Check sheet for the modelled part. Datum: model origin and axes. Units: mm. Face numbers are marked on the shaded views. A direction names the side the tool comes from. Round coordinates to 2 decimals unless told otherwise and drop trailing zeros. Write each loop counter-clockwise with the first axis right and the second up, starting at its lowest first coordinate (ties: lowest second). Pieces come first, ordered by that corner, then holes. Notation, with made-up numbers: (86, 52.5) -> (140, 52.5) arc R17 ccw to (140, 81.5) -> close; hole circle Ø7 at (-3.75, -13.5). An arc over 180 degrees is marked (long way). One line per item, written item: value.
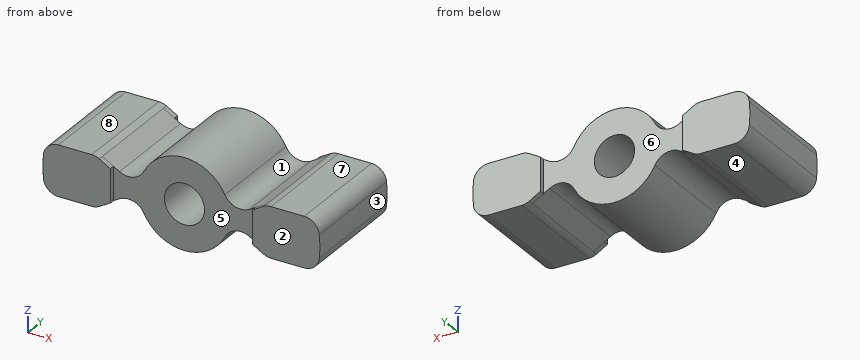
from build123d import *

# Parameters (mm, degrees)
F0_R     = 4
F1_DEPTH = 10
F3_DEPTH = 1


# Not quite as in the source:
# - a pattern or mirror of a feature is missing from the dataset's text; its kind, count and spacing are read off the source's solid


with BuildPart() as f1:
    # F0 (on Front) → F1 (new body, symmetric)
    with BuildSketch(Plane.XZ):
        with BuildLine():
            ThreePointArc((-12.8973712231, -2.6245379145), (-10.1504183848, -2.3006178802), (-8.0261072806, -4.072051316))
            ThreePointArc((-8.0261072806, -4.072051316), (0, -9), (8.0261072806, -4.072051316))
            ThreePointArc((8.0261072806, -4.072051316), (10.1504183848, -2.3006178802), (12.8973712231, -2.6245379145))
            Line((12.8973712231, -2.6245379145), (16.315639824, -4.5980762114))
            ThreePointArc((16.315639824, -4.5980762114), (17.0391826887, -4.8977774789), (17.815639824, -5))
            Line((17.815639824, -5), (24.4182308941, -5))
            ThreePointArc((24.4182308941, -5), (26.4511236757, -4.2062064588), (27.4082183506, -2.2448979592))
            ThreePointArc((27.4082183506, -2.2448979592), (27.5, 0), (27.4082183506, 2.2448979592))
            ThreePointArc((27.4082183506, 2.2448979592), (26.4511236757, 4.2062064588), (24.4182308941, 5))
            Line((24.4182308941, 5), (17.815639824, 5))
            ThreePointArc((17.815639824, 5), (17.0391826887, 4.8977774789), (16.315639824, 4.5980762114))
            Line((16.315639824, 4.5980762114), (12.8973712231, 2.6245379145))
            ThreePointArc((12.8973712231, 2.6245379145), (10.1504183848, 2.3006178802), (8.0261072806, 4.072051316))
            ThreePointArc((8.0261072806, 4.072051316), (0, 9), (-8.0261072806, 4.072051316))
            ThreePointArc((-8.0261072806, 4.072051316), (-10.1504183848, 2.3006178802), (-12.8973712231, 2.6245379145))
            Line((-12.8973712231, 2.6245379145), (-16.315639824, 4.5980762114))
            ThreePointArc((-16.315639824, 4.5980762114), (-17.0391826887, 4.8977774789), (-17.815639824, 5))
            Line((-17.815639824, 5), (-24.4182308941, 5))
            ThreePointArc((-24.4182308941, 5), (-26.4511236757, 4.2062064588), (-27.4082183506, 2.2448979592))
            ThreePointArc((-27.4082183506, 2.2448979592), (-27.5, 0), (-27.4082183506, -2.2448979592))
            ThreePointArc((-27.4082183506, -2.2448979592), (-26.4511236757, -4.2062064588), (-24.4182308941, -5))
            Line((-24.4182308941, -5), (-17.815639824, -5))
            ThreePointArc((-17.815639824, -5), (-17.0391826887, -4.8977774789), (-16.315639824, -4.5980762114))
            Line((-16.315639824, -4.5980762114), (-12.8973712231, -2.6245379145))
        make_face()
        Circle(F0_R, mode=Mode.SUBTRACT)
    extrude(amount=F1_DEPTH, both=True)

    # F2 (on face) → F3 (join)
    with BuildSketch(Plane.XZ.offset(10)):
        with BuildLine():
            Line((-24.4182308941, -5), (-17.815639824, -5))
            ThreePointArc((-17.815639824, -5), (-17.0391826887, -4.8977774789), (-16.315639824, -4.5980762114))
            Line((-16.315639824, -4.5980762114), (-14.1075365245, -3.323227177))
            Line((-14.1075365245, -3.323227177), (-14.1075365245, 3.323227177))
            Line((-14.1075365245, 3.323227177), (-16.315639824, 4.5980762114))
            ThreePointArc((-16.315639824, 4.5980762114), (-17.0391826887, 4.8977774789), (-17.815639824, 5))
            Line((-17.815639824, 5), (-24.4182308941, 5))
            ThreePointArc((-24.4182308941, 5), (-26.4511236757, 4.2062064588), (-27.4082183506, 2.2448979592))
            ThreePointArc((-27.4082183506, 2.2448979592), (-27.5, 0), (-27.4082183506, -2.2448979592))
            ThreePointArc((-27.4082183506, -2.2448979592), (-26.4511236757, -4.2062064588), (-24.4182308941, -5))
        make_face()
        with BuildLine():
            Line((14.1075365245, -3.323227177), (16.315639824, -4.5980762114))
            ThreePointArc((16.315639824, -4.5980762114), (17.0391826887, -4.8977774789), (17.815639824, -5))
            Line((17.815639824, -5), (24.4182308941, -5))
            ThreePointArc((24.4182308941, -5), (26.4511236757, -4.2062064588), (27.4082183506, -2.2448979592))
            ThreePointArc((27.4082183506, -2.2448979592), (27.5, 0), (27.4082183506, 2.2448979592))
            ThreePointArc((27.4082183506, 2.2448979592), (26.4511236757, 4.2062064588), (24.4182308941, 5))
            Line((24.4182308941, 5), (17.815639824, 5))
            ThreePointArc((17.815639824, 5), (17.0391826887, 4.8977774789), (16.315639824, 4.5980762114))
            Line((16.315639824, 4.5980762114), (14.1075365245, 3.323227177))
            Line((14.1075365245, 3.323227177), (14.1075365245, -3.323227177))
        make_face()
    f3 = extrude(amount=F3_DEPTH)

    # F3_copies: F3 across plane
    add(f3.mirror(Plane.ZX))


solid = f1.part
Item 1: Sectioned sample at B-B on z = 0. Enter the section's corners in (x, y).
Answer:
outline: (-27.5, -11) -> (-14.11, -11) -> (-14.11, -10) -> (-4, -10) -> (-4, 10) -> (-14.11, 10) -> (-14.11, 11) -> (-27.5, 11) -> close; (4, -10) -> (14.11, -10) -> (14.11, -11) -> (27.5, -11) -> (27.5, 11) -> (14.11, 11) -> (14.11, 10) -> (4, 10) -> close
Item 2: Sectioned sample at D-D on x = 17. Enter the section's corners in (y, z).
Answer:
outline: (-11, -4.89) -> (11, -4.89) -> (11, 4.89) -> (-11, 4.89) -> close
Item 3: Thickness scan on line 1 (X direction, y = -7, z = 4.75); line 2 (X direction, y = 5, z = -3.5); line 3 (Y direction, x = 8, z = -3). Record the ranges inside material, lowest first.
Answer:
line 1: x = -25.62 to -16.62, -7.64 to 7.64, 16.62 to 25.62
line 2: x = -27.02 to -14.41, -8.39 to -1.94, 1.94 to 8.39, 14.41 to 27.02
line 3: y = -10 to 10
Item 4: Sectioned sample at C-C on y = 1.25. Enter the section's corners in (x, z).
Answer:
outline: (-27.41, -2.24) arc R3 ccw to (-24.42, -5) -> (-17.82, -5) arc R3 ccw to (-16.32, -4.6) -> (-12.9, -2.62) arc R3.5 cw to (-8.03, -4.07) arc R9 ccw to (8.03, -4.07) arc R3.5 cw to (12.9, -2.62) -> (16.32, -4.6) arc R3 ccw to (17.82, -5) -> (24.42, -5) arc R3 ccw to (27.41, -2.24) arc R27.5 ccw to (27.41, 2.24) arc R3 ccw to (24.42, 5) -> (17.82, 5) arc R3 ccw to (16.32, 4.6) -> (12.9, 2.62) arc R3.5 cw to (8.03, 4.07) arc R9 ccw to (-8.03, 4.07) arc R3.5 cw to (-12.9, 2.62) -> (-16.32, 4.6) arc R3 ccw to (-17.82, 5) -> (-24.42, 5) arc R3 ccw to (-27.41, 2.24) arc R27.5 ccw to start; hole circle Ø8 at (0, 0)
Item 5: Depth check by flat-ended pin: P1, Ø10, axis at x = 22, y = 5.5, coming from the -Z side; P2, Ø1.1, axis at y = 10.5, z = -1, coming from the -X side; P3, Ø5.5, axis at x = -20, y = -4.5, coming from the +Z side. Enter the tip coordinate at first touch or a pass-through.
Answer:
P1: stops at z = -5
P2: stops at x = -27.5
P3: stops at z = 5
Item 6: Sectioned sample at A-A on x = 0. Enter the section's corners in (y, z).
Answer:
outline: (-10, -9) -> (10, -9) -> (10, -4) -> (-10, -4) -> close; (-10, 4) -> (10, 4) -> (10, 9) -> (-10, 9) -> close
Item 7: Mould release check, pull along X, two halves, no side actions. Record for the marked faces 1, 2 and 3: pulls with the +X half, pulls with the -X half, needs draft (parallel to the pull), parting line crosses it, or undercut.
Answer:
face 1: undercut
face 2: needs draft
face 3: pulls with the +X half
Item 8: Tool access check on the marked faces 4, 5, 6, 7 and 8. Record the directions out of +Z, -Z, +X, -X, +Y, -Y that give a thin tool (end or side, any length) a straight path to the whole face; none if there is none.
Answer:
face 4: -Z, -X, +Y, -Y
face 5: +Z, -Z, -Y
face 6: +Z, -Z, +Y
face 7: +Z, +X, +Y, -Y
face 8: +Z, -X, +Y, -Y
